The figure shows three views and two pictorial views of one solid part (mm, origin at its lowest corner). Answer the questions. A direction names the side the tool comes from. Give positions to 0.01 mm unless a question says otherwise; leave off trailing zeros. Order: outer loops, then holes, each group sorted by start corner. A loop starts at its lowest first (then second) coordinate and runs counter-clockwise, first axis right, second up. Notation, with made-up numbers: M -5,-33.5 L 39,-33.5 A32 ccw 39,-1.5 Z; hole C 23.25,28 d3. An arc over 180 degrees is marked long. One line per item, written item: value.
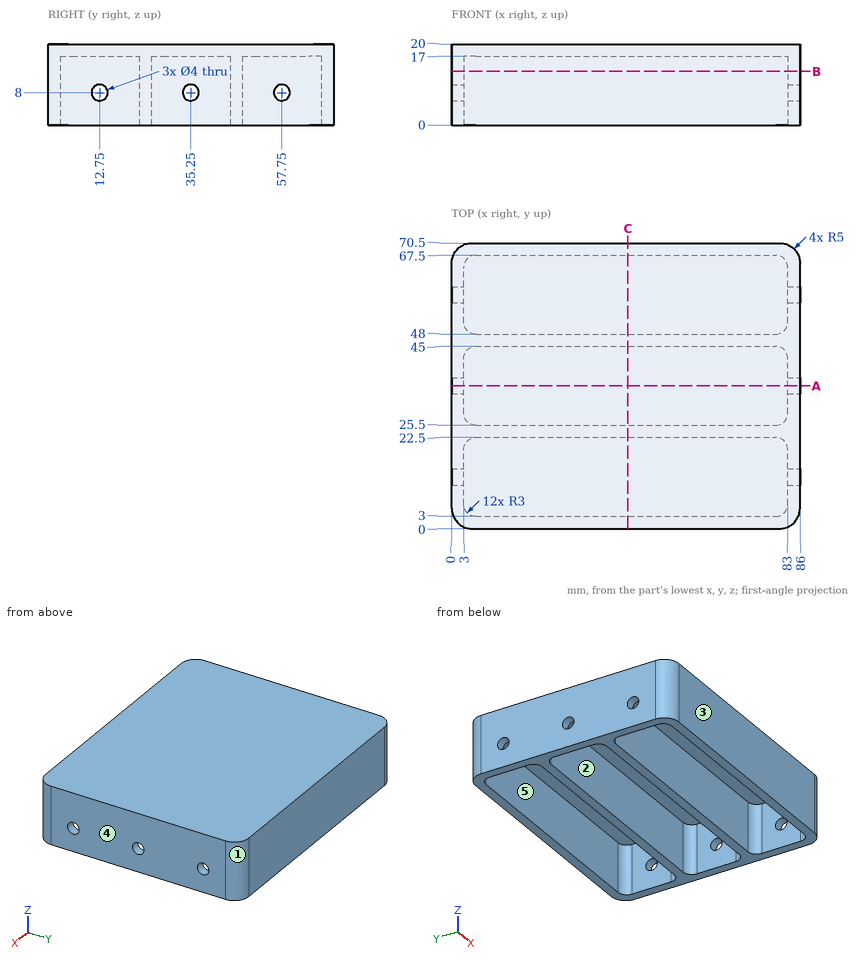
1) Determine the mould class of the marked faces 3, 4 and 5 for opening direction X: +X half, -X half, draft (parallel to the pull), parting line (faces both ways), or undercut.
Reported:
face 3: draft
face 4: +X half
face 5: undercut
2) Consider probe 1 along Y at (x, z) = (12, 3); probe 2 along Z at (x, y) = (1, 35); probe 3 along X at (y, z) = (15, 16). Determine where each line is inside the solid, lowest interval first.
Reported:
probe 1: y = 0 to 3, 22.5 to 25.5, 45 to 48, 67.5 to 70.5
probe 2: z = 0 to 6.02, 9.98 to 20
probe 3: x = 0 to 3, 83 to 86
3) Find section A-A, the plane y = 35.25. Write down the section's boundary in (x, z).
Reported:
outline: M 0,0 L 3,0 L 3,6 L 0,6 Z; M 0,10 L 3,10 L 3,17 L 83,17 L 83,10 L 86,10 L 86,20 L 0,20 Z; M 83,0 L 86,0 L 86,6 L 83,6 Z
4) Find section B-B, the plane z = 13.25. Count the separate pieces of the cut face and the enclosed holes in it, plus the area to 3 significant figures.
Reported:
separate pieces: 1
enclosed holes: 3
area: 1,380 mm^2
5) Find section C-C, the plane x = 43.5. Write down the section's boundary in (y, z).
Reported:
outline: M 0,0 L 3,0 L 3,17 L 22.5,17 L 22.5,0 L 25.5,0 L 25.5,17 L 45,17 L 45,0 L 48,0 L 48,17 L 67.5,17 L 67.5,0 L 70.5,0 L 70.5,20 L 0,20 Z
6) This flat-tipped pin is pushed along its axis until it touches: pin 1 Ø15.5 at (x, y) = (35, 37) entering from -Z. Where does it stop, or does it pass through?
Reported:
pin 1: stops at z = 17
7) Which of the six approach directions +Z, -Z, +X, -X, +Y, -Y give full straight-line access (tool end or side, diameter ignored) to the marked faces 1 and 2?
Reported:
face 1: +Z, -Z, +X, +Y
face 2: -Z
